Design review of the part built by this model. Coordinates are the model's own, in mm. Round coordinates to 2 decimals unless told otherwise and drop trailing zeros. Order: outer loops, then holes, each group sorted by start corner. A loop starts at its lowest first (then second) coordinate and runs counter-clockwise, first axis right, second up. Notation, with made-up numbers: (21.25, 72.25) - (80.25, 72.25) arc R21 ccw to (80.25, 95.25) - close; hole circle Ø4 at (-27.5, -40). An arc over 180 degrees is marked (long way). Write item = value, one per line.
from build123d import *

# Parameters (mm, degrees)
BOSS_EXTRUDE1_DEPTH = 1.5875
CUT_EXTRUDE5_DEPTH  = 1733.843331241


with BuildPart() as part:
    # Sketch3 → Boss-Extrude1 (new, symmetric)
    with BuildSketch(Plane(origin=(0, 0, 0), x_dir=(0, 0, -1), z_dir=(1, 0, 0))):
        with BuildLine():
            Line((1727.2, -139.7), (1727.2, 0))
            Line((1727.2, 0), (1643.3038, 0.398291906))
            Line((1643.3038, 0.398291906), (1643.3038, -13.081))
            Line((1643.3038, -13.081), (1617.1418, -13.081))
            Line((1617.1418, -13.081), (1617.1418, 0.522494347))
            Line((1617.1418, 0.522494347), (1346.2, 1.808773415))
            Line((1346.2, 1.808773415), (1346.2, -99.791226585))
            Line((1346.2, -99.791226585), (1342.6186, -99.791226585))
            Line((1342.6186, -99.791226585), (1342.6186, 1.825775885))
            Line((1342.6186, 1.825775885), (1148.0038, 2.749697345))
            Line((1148.0038, 2.749697345), (1148.0038, -13.081))
            Line((1148.0038, -13.081), (1121.8418, -13.081))
            Line((1121.8418, -13.081), (1121.8418, 2.873899787))
            Line((1121.8418, 2.873899787), (1020.6228, 3.35443059))
            Line((1020.6228, 3.35443059), (1020.6228, -98.24556941))
            Line((1020.6228, -98.24556941), (1017.0414, -98.24556941))
            Line((1017.0414, -98.24556941), (1017.0414, 3.371433061))
            Line((1017.0414, 3.371433061), (918.828185443, 3.837694088))
            ThreePointArc((918.828185443, 3.837694088), (919.259095992, 1.94031106), (919.4038, 0))
            ThreePointArc((919.4038, 0), (904.32109725, -12.926938814), (893.85441584, 3.956255481))
            Line((893.85441584, 3.956255481), (807.550680013, 4.365977011))
            Line((807.550680013, 4.365977011), (525.3228, -14.277479423))
            Line((525.3228, -14.277479423), (525.3228, -103.177479423))
            Line((525.3228, -103.177479423), (521.7414, -103.177479423))
            Line((521.7414, -103.177479423), (521.7414, -14.514060143))
            Line((521.7414, -14.514060143), (260.820750269, -31.75))
            Line((260.820750269, -31.75), (222.61445683, -31.75))
            ThreePointArc((222.61445683, -31.75), (209.7532, -42.4434), (196.89194317, -31.75))
            Line((196.89194317, -31.75), (-69.6468, -31.75))
            Line((-69.6468, -31.75), (-69.6468, -107.95))
            Line((-69.6468, -107.95), (-73.2282, -107.95))
            Line((-73.2282, -107.95), (-73.2282, -31.75))
            Line((-73.2282, -31.75), (-311.45864317, -31.75))
            ThreePointArc((-311.45864317, -31.75), (-324.3199, -42.4434), (-337.18115683, -31.75))
            Line((-337.18115683, -31.75), (-399.579249731, -31.75))
            Line((-399.579249731, -31.75), (-399.579249731, 66.658263044))
            Line((-399.579249731, 66.658263044), (-449.685071474, 66.658263044))
            ThreePointArc((-449.685071474, 66.658263044), (-462.454755632, 56.414114736), (-475.224439789, 66.658263044))
            Line((-475.224439789, 66.658263044), (-512.373001058, 66.658263044))
            Line((-512.373001058, 66.658263044), (-559.824848458, -29.3624))
            Line((-559.824848458, -29.3624), (-571.9699, -29.3624))
            Line((-571.9699, -29.3624), (-571.9699, -105.5624))
            Line((-571.9699, -105.5624), (-575.5513, -105.5624))
            Line((-575.5513, -105.5624), (-575.5513, -29.3624))
            Line((-575.5513, -29.3624), (-672.719, -29.3624))
            Line((-672.719, -29.3624), (-672.719, -42.4434))
            Line((-672.719, -42.4434), (-698.881, -42.4434))
            Line((-698.881, -42.4434), (-698.881, -29.3624))
            Line((-698.881, -29.3624), (-762, -29.3624))
            Line((-762, -29.3624), (-762, -139.7))
            Line((-762, -139.7), (1727.2, -139.7))
        make_face()
    extrude(amount=BOSS_EXTRUDE1_DEPTH, both=True)

    # Sketch5 → Cut-Extrude5 (cut, through all)
    with BuildSketch(Plane(origin=(1.5875, 0, 0), x_dir=(0, 0, -1), z_dir=(1, 0, 0))):
        Polygon((1310.5638, -22.728682836), (1310.5638, 1.977954022), (1164.5138, 2.671317164), (1164.5138, -22.728682836), align=None)
        Polygon((120.8532, -44.45), (-31.5468, -42.857236965), (-31.5468, -31.75), (120.8532, -31.75), align=None)
    extrude(amount=-CUT_EXTRUDE5_DEPTH, mode=Mode.SUBTRACT)


solid = part.part
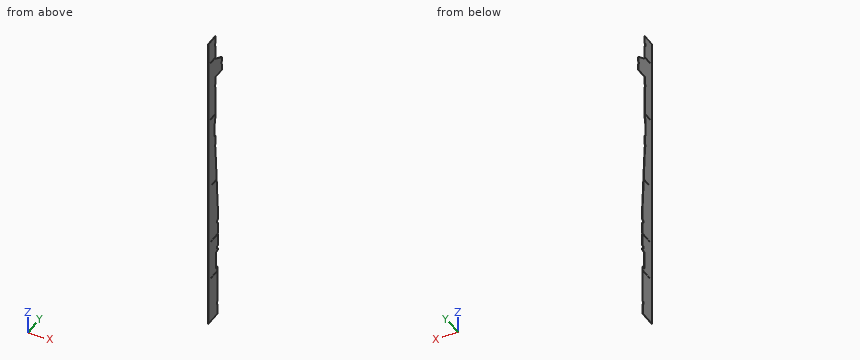
1) To check wall thickness, follow L1, parallel to Z at x = 0.6, y = -76; L2, parallel to Y at x = 1.45, z = -243; L3, parallel to Y at x = -0.35, z = -1256.5. State the ranges of each line that lie inside material, in increasing order. Write a range as from..to.
Findings:
L1 = -1727.2..-1346.2, -1342.62..-1020.62, -1017.04..-525.32, -521.74..69.65, 73.23..571.97, 575.55..762
L2 = -139.7..-31.75
L3 = -139.7..-22.73
2) We need section A-A on z = -393. Write out the cut boundary in (x, y), and give its area (3 significant figures).
Findings:
outline = (-1.59, -139.7) - (1.59, -139.7) - (1.59, -23.02) - (-1.59, -23.02) - close
area = 370 mm^2
3) Clearance check with flat-ended pins moving along their axes: pin 1 Ø1 at (x, z) = (0.5, 71.5) entering from +Y; pin 2 Ø1.6 at (x, z) = (-0.5, -1631.5) entering from +Y; pin 3 Ø1 at (x, y) = (0, -7) entering from +Z. State where each tip first meets the part, or that it passes through.
Findings:
pin_1 = -107.95
pin_2 = -13.08
pin_3 = 549.02
